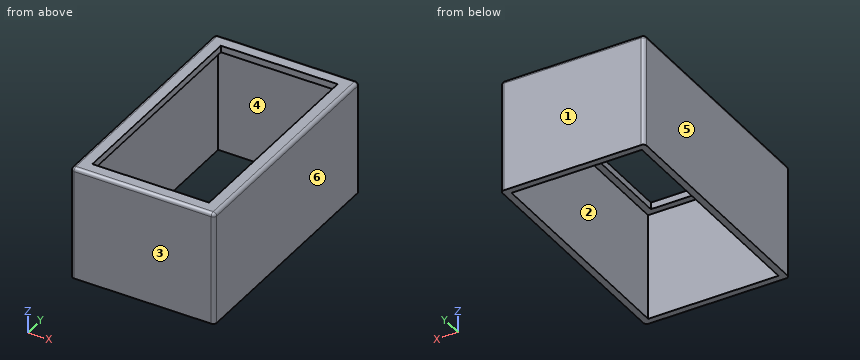
from build123d import *

# Parameters (mm, degrees)
SKETCH1_W           = 10.7315
SKETCH1_H           = 18.034
BOSS_EXTRUDE1_DEPTH = 7.9375
SHELL1_T            = -0.508
SKETCH2_W           = 10.7315
SKETCH2_H           = 18.034
SKETCH2_W_2         = 8.6995
SKETCH2_H_2         = 16.002
EXTRUDE_THIN1_DEPTH = 0.508
FILLET2_R           = 0.254


with BuildPart() as part:
    # Sketch1 → Boss-Extrude1 (new body)
    with BuildSketch(Plane.XY):
        with Locations((14.669644351, 41.878696913)):
            Rectangle(SKETCH1_W, SKETCH1_H)
    extrude(amount=BOSS_EXTRUDE1_DEPTH)

    # Shell1
    shell1_openings = [part.faces().sort_by_distance(p)[0] for p in [
        (14.669644351, 41.878696913, 7.9375),
        (14.669644351, 41.878696913, 0),
    ]]
    offset(amount=SHELL1_T, openings=shell1_openings, kind=Kind.INTERSECTION)

    # Sketch2 → Extrude-Thin1 (add)
    with BuildSketch(Plane.XY.offset(7.9375)):
        with Locations((14.669644351, 41.878696913)):
            Rectangle(SKETCH2_W, SKETCH2_H)
        with Locations((14.669644351, 41.878696913)):
            Rectangle(SKETCH2_W_2, SKETCH2_H_2, mode=Mode.SUBTRACT)
    extrude(amount=EXTRUDE_THIN1_DEPTH)

    # Fillet2
    fillet2_edges = [part.edges().sort_by_distance(p)[0] for p in [
        (14.669644351, 32.861696913, 8.4455),
        (20.035394351, 41.878696913, 8.4455),
        (14.669644351, 50.895696913, 8.4455),
        (9.303894351, 41.878696913, 8.4455),
        (9.303894351, 50.895696913, 4.22275),
        (20.035394351, 50.895696913, 4.22275),
        (20.035394351, 32.861696913, 4.22275),
        (9.303894351, 32.861696913, 4.22275),
    ]]
    fillet(fillet2_edges, radius=FILLET2_R)


solid = part.part
Geometry check sheet. Reference: the model listing, model coordinates, mm. Face numbers are marked on the shaded views. A direction names the side the tool comes from. Give positions to 0.01 mm unless a question says otherwise; leave off trailing zeros. Order: outer loops, then holes, each group sorted by start corner. A loop starts at its lowest first (then second) coordinate and runs counter-clockwise, first axis right, second up. Notation, with made-up numbers: M -24.75,-15 L -15.75,-15 A21 cw -15.75,20 Z; hole C -25,-33 d2. An arc over 180 degrees is marked long. Use a Markdown table: item, result.
Item 1: Section check C-C (x = 10.75). Record the cut outline in (y, z), and give its area (3 significant figures).
Answers follow:
| item | result |
|---|---|
| outline | M 32.86,0 L 33.37,0 L 33.37,7.94 L 33.88,7.94 L 33.88,8.45 L 33.12,8.45 A0.25 ccw 32.86,8.19 Z; M 49.88,7.94 L 50.39,7.94 L 50.39,0 L 50.9,0 L 50.9,8.19 A0.25 ccw 50.64,8.45 L 49.88,8.45 Z |
| area | 9.07 mm2 |
Item 2: Material ranges on line 1 along Y through (x, z) = (11.75, 3.5); line 2 along X through (y, z) = (41.75, 1.75); line 3 along Y through (x, z) = (13.25, 8), recorded low to high.
Answers follow:
| item | result |
|---|---|
| line 1 | y = 32.86 to 33.37, 50.39 to 50.9 |
| line 2 | x = 9.3 to 9.81, 19.53 to 20.04 |
| line 3 | y = 32.86 to 33.88, 49.88 to 50.9 |
Item 3: Section check B-B (z = 4.5). Record the cut outline in (x, y), and give its area (3 significant figures).
Answers follow:
| item | result |
|---|---|
| outline | M 9.3,33.12 A0.25 ccw 9.56,32.86 L 19.78,32.86 A0.25 ccw 20.04,33.12 L 20.04,50.64 A0.25 ccw 19.78,50.9 L 9.56,50.9 A0.25 ccw 9.3,50.64 Z; hole M 9.81,33.37 L 19.53,33.37 L 19.53,50.39 L 9.81,50.39 Z |
| area | 28.1 mm2 |
Item 4: Section check A-A (y = 35.5). Record the cut outline in (x, z).
Answers follow:
| item | result |
|---|---|
| outline | M 9.3,0 L 9.81,0 L 9.81,7.94 L 10.32,7.94 L 10.32,8.45 L 9.56,8.45 A0.25 ccw 9.3,8.19 Z; M 19.02,7.94 L 19.53,7.94 L 19.53,0 L 20.04,0 L 20.04,8.19 A0.25 ccw 19.78,8.45 L 19.02,8.45 Z |
Item 5: Tool access check on the marked faces 1 and 2. Record the directions out of +Z, -Z, +X, -X, +Y, -Y that give a thin tool (end or side, any length) a straight path to the whole face; none if there is none.
Answers follow:
| item | result |
|---|---|
| face 1 | +Z, -Z, +X, -X, +Y |
| face 2 | -Z |
Item 6: Draft check along X on the marked faces 3, 4, 5 and 6. Enter one of: +X half, -X half, draft (parallel to the pull), parting line (faces both ways), or undercut.
Answers follow:
| item | result |
|---|---|
| face 3 | draft |
| face 4 | undercut |
| face 5 | -X half |
| face 6 | +X half |
